```python
from build123d import *

# Parameters (mm, degrees)
SKETCH1_W               = 30
SKETCH1_H               = 60
BOSS_EXTRUDE1_DEPTH     = 287.5
SKETCH2_R               = 10.5
CUT_EXTRUDE1_DEPTH      = 295.076945713
SKETCH3_R               = 5.1
CUT_EXTRUDE2_DEPTH      = 10
SKETCH4_R               = 4
SKETCH4_R_2             = 1.75
CUT_EXTRUDE3_DEPTH      = 295.076945713
SKETCH5_R               = 2
CUT_EXTRUDE4_DEPTH      = 7
MIRROR1_COPY_1_SKETCH_R = 5.1
MIRROR1_COPY_1_DEPTH    = 10


with BuildPart() as part:
    # Sketch1 → Boss-Extrude1 (new, symmetric)
    with BuildSketch(Plane.XY):
        Rectangle(SKETCH1_W, SKETCH1_H)
    extrude(amount=BOSS_EXTRUDE1_DEPTH, both=True)

    # Sketch2 → Cut-Extrude1 (cut, through all)
    with BuildSketch(Plane(origin=(0, 30, 0), x_dir=(1, 0, 0), z_dir=(0, 1, 0))):
        with Locations((15, -262.5)):
            Circle(SKETCH2_R)
    cut_extrude1 = extrude(amount=-CUT_EXTRUDE1_DEPTH, mode=Mode.SUBTRACT)

    # Sketch3 → Cut-Extrude2 (cut)
    with BuildSketch(Plane(origin=(0, 30, 0), x_dir=(1, 0, 0), z_dir=(0, 1, 0))):
        with Locations(Location((0, -237.5, 0), (0, 0, 270))):
            Circle(SKETCH3_R)
    cut_extrude2 = extrude(amount=-CUT_EXTRUDE2_DEPTH, mode=Mode.SUBTRACT)

    # Mirror2: Cut-Extrude2 across plane
    add(cut_extrude2.mirror(Plane.ZX), mode=Mode.SUBTRACT)

    # Sketch4 → Cut-Extrude3 (cut, through all)
    with BuildSketch(Plane(origin=(0, 30, 0), x_dir=(1, 0, 0), z_dir=(0, 1, 0))):
        with Locations(Location((0, -237.5, 0), (0, 0, 270))):
            Circle(SKETCH4_R)
        with Locations(Location((-8, -237.5, 0), (0, 0, 270))):
            Circle(SKETCH4_R_2)
        with Locations(Location((0, -229.5, 0), (0, 0, 270))):
            Circle(SKETCH4_R_2)
        with Locations(Location((8, -237.5, 0), (0, 0, 270))):
            Circle(SKETCH4_R_2)
        with Locations(Location((0, -245.5, 0), (0, 0, 270))):
            Circle(SKETCH4_R_2)
    cut_extrude3 = extrude(amount=-CUT_EXTRUDE3_DEPTH, mode=Mode.SUBTRACT)

    # Sketch5 → Cut-Extrude4 (cut)
    with BuildSketch(Plane(origin=(15, 0, 0), x_dir=(0, 0, -1), z_dir=(1, 0, 0))):
        with Locations((-246, 24.5)):
            Circle(SKETCH5_R)
        with Locations((-246, 5)):
            Circle(SKETCH5_R)
        with Locations(Location((-246, -5, 0), (0, 0, 180))):
            Circle(SKETCH5_R)
        with Locations(Location((-246, -24.5, 0), (0, 0, 180))):
            Circle(SKETCH5_R)
    cut_extrude4 = extrude(amount=-CUT_EXTRUDE4_DEPTH, mode=Mode.SUBTRACT)

    # Mirror1: Cut-Extrude1, Cut-Extrude2, Cut-Extrude3, Cut-Extrude4 across plane
    add(cut_extrude1.mirror(Plane.XY), mode=Mode.SUBTRACT)
    add(cut_extrude2.mirror(Plane.XY), mode=Mode.SUBTRACT)
    add(cut_extrude3.mirror(Plane.XY), mode=Mode.SUBTRACT)
    add(cut_extrude4.mirror(Plane.XY), mode=Mode.SUBTRACT)

    # Mirror1 copy 1 sketch → Mirror1 copy 1 (cut)
    with BuildSketch(Plane.XZ.offset(30)):
        with Locations(Location((0, -237.5, 0), (0, 0, 270))):
            Circle(MIRROR1_COPY_1_SKETCH_R)
    extrude(amount=-MIRROR1_COPY_1_DEPTH, mode=Mode.SUBTRACT)


solid = part.part
```
Geometry check sheet. Reference: the model listing, model coordinates, mm. A direction names the side the tool comes from. Coordinates: 2 decimals unless noted, no trailing zeros.
Item 1: Mould release check, pull along X, two halves, no side actions. Record for faces 4 (the flat face through (0, 30, 4)), 5 (the flat face through (15, 0, 280)), 6 (the cylindrical face through (1.532, 25.07, 242.364)), 7 (the flat face through (-15, 0, 4)): released by +X, released by -X, zero draft, split by the parting line, or undercut.
Item 2: Scan lines: line 1 along X through (y, z) = (-23.5, 237.5); line 2 along Y through (x, z) = (10.75, 246); line 3 along X through (y, z) = (-5.5, 245.5). Record each from-to range of solid material in increasing order.
Item 3: Section check A-A (y = -14). Count the separate pieces of the cut face and the enclosed holes in it, plus the area to 3 significant figures.
Item 4: Depth check by flat-ended pin: pin 1 (6 mm diameter, centred on x = 0, z = -237.5, fed in from +Y). Enter the tip coordinate at first touch or a pass-through.
Item 5: Tool access check on faces 1 (the flat face through (0, 0, 287.5)), 2 (the cylindrical face through (1.532, 25.07, -242.364)), 3 (the flat face through (-3, -20, 234)). Record the directions out of +Z, -Z, +X, -X, +Y, -Y that give a thin tool (end or side, any length) a straight path to the whole face; none if there is none.
Check sheet entries:
1. face 4: zero draft
1. face 5: released by +X
1. face 6: undercut
1. face 7: released by -X
2. line 1: x = -15 to -9.75, -6.25 to -5.1, 5.1 to 6.25, 9.75 to 15
2. line 2: y = -30 to -26.5, -22.5 to -7, -3 to 3, 7 to 22.5, 26.5 to 30
2. line 3: x = -15 to -1.75, 1.75 to 8
3. separate pieces: 1
3. enclosed holes: 10
3. area: 16,700 mm2
4. pin 1: passes through
5. face 1: +Z, +X, -X, +Y, -Y
5. face 2: +Y
5. face 3: -Y
